Autodesk Inventor part; units mm, degrees
ref_plane "YZ Plane" through (0, 0, 0) normal (1, 0, 0) x (0, 1, 0)
ref_plane "XZ Plane" through (0, 0, 0) normal (0, 1, 0) x (-1, 0, 0)
ref_plane "XY Plane" through (0, 0, 0) normal (0, 0, 1) x (1, 0, 0)
sketch "Sketch1" plane through (0, 0, 0) normal (0, 0, 1) x (1, 0, 0)
  line L0 (0, 0) -> (0, 13.4062)
  line L1 (0, 0) -> (20.3742, 0)
  circle A0 centre (9.525, 12.7) radius 9.525 construction
  circle A1 centre (9.525, 12.7) radius 3.2004
  line L2 (31.75, 0) -> (7.8407, 6.5775)
  arc A2 (3.3908, 14.3415) -> (7.8407, 6.5775) centre (9.525, 12.7) ccw
  line L3 (31.75, 0) -> (76.2, 0)
  line L4 (76.2, 0) -> (76.2, 25.4)
  line L5 (76.2, 25.4) -> (31.75, 25.4)
  line L6 (31.75, 25.4) -> (31.75, 57.15)
  line L7 (31.75, 57.15) -> (19.05, 57.15)
  line L8 (19.05, 57.15) -> (19.05, 69.85)
  line L9 (19.05, 69.85) -> (6.35, 69.85)
  line L10 (6.35, 69.85) -> (6.35, 25.4)
  line L11 (6.35, 25.4) -> (3.3908, 14.3415)
  circle A3 centre (12.7, 63.5) radius 2.4892
  line L12 (12.7, 69.85) -> (12.7, 63.5)
  circle A4 centre (44.45, 12.7) radius 2.4892
  circle A5 centre (57.15, 12.7) radius 2.4892
  circle A6 centre (69.85, 12.7) radius 2.4892
  circle A7 centre (19.05, 38.1) radius 2.4892
  circle A8 centre (19.05, 50.8) radius 2.4892
  line L13 (19.05, 50.8) -> (19.05, 38.1) construction
  arc A9 (31.75, 29.8901) -> (36.2401, 25.4) centre (33.9951, 27.6451) ccw
  circle A10 centre (31.2867, 27.5124) radius 0.4633 construction
  circle A11 centre (33.8624, 24.9367) radius 0.4633 construction
  line L14 (31.75, 25.4) -> (31.2867, 27.5124) construction
  line L15 (31.75, 25.4) -> (33.8624, 24.9367) construction
  point P0 (76.2, 12.7)
  dimension "d0" = 19.05
  dimension "d1" = 3.175
  dimension "d2" = 6.4008
  dimension "d6" = 12.7
  dimension "d7" = 25.4
  dimension "d8" = 4.9784
  dimension "d16" = 6.35
  dimension "d17" = 25.4
  dimension "d19" = 6.35
  dimension "d24" = 12.7
  dimension "d29" = 6.35
  dimension "d30" = 12.7
  dimension "d35" = 12.7
  dimension "d36" = 12.7
  dimension "d37" = 12.7
  dimension "d38" = 6.35
  dimension "d39" = 12.7
  dimension "d40" = 6.35
extrude "Extrusion1" add sketch "Sketch1" along normal blind 3.175 contours L2 A2 L11 L10 L9 L8 L7 L6 A9 L5 L4 L3
fillet "Fillet1" radius 3.175 8 edges at (6.35, 69.85, 1.5875) (19.05, 69.85, 1.5875) (76.2, 25.4, 1.5875) (76.2, 0, 1.5875) (6.35, 25.4, 1.5875) (31.75, 0, 1.5875) (31.75, 57.15, 1.5875) (19.05, 57.15, 1.5875)
equation "\"d24\" = d11"
properties part number "Bottom Bearing Plate (R4 - 0.25in Between Stages)" material "Aluminum 6061"
Work out the finished part from the listing and answer in its coordinate system (mm). A direction names the side the tool comes from. Coordinates: 2 decimals unless noted, no trailing zeros. Write each loop counter-clockwise with the first axis right and the second up, starting at its lowest first coordinate (ties: lowest second). Pieces come first, ordered by that corner, then holes. Notation, with made-up numbers: M -6,87.25 L 1,87.25 A22 ccw 1,106.25 Z; hole C 46.25,73.5 d8. An arc over 180 degrees is marked long. Write item = value, one per line.
1. The part is cut by section D-D (y = 45). Determine the outline of the cut face in (x, z) (3 decimals).
Solution:
outline = M 6.35,0 L 31.75,0 L 31.75,3.175 L 6.35,3.175 Z
2. The part is cut by section A-A (y = 63.5). Determine the outline of the cut face in (x, z) (3 decimals).
Solution:
outline = M 6.35,0 L 10.211,0 L 10.211,3.175 L 6.35,3.175 Z; M 15.189,0 L 19.05,0 L 19.05,3.175 L 15.189,3.175 Z
3. For faces 1 (the face through (6.35, 47, 2)), 2 (the face through (55, 25.4, 2)), 3 (the face through (18.51, 53.23, 1.57)), determine the directions among +Z, -Z, +X, -X, +Y, -Y from which every point of the face is accessible in a straight line to the end or side of a thin tool.
Solution:
face_1 = +Z, -Z, -X, +Y
face_2 = +Z, -Z, +X, +Y
face_3 = +Z, -Z
4. Determine the mould class of faces 4 (the face through (19.05, 63, 2)), 5 (the face through (9.108, 9.527, 1.565)), 6 (the face through (25, 57.15, 2)) for opening direction Y: released by +Y, released by -Y, zero draft, split by the parting line, or undercut.
Solution:
face_4 = zero draft
face_5 = undercut
face_6 = released by +Y
5. Flat-ended cylindrical pins translate along their axes: pin 1 (1 mm diameter, centred on y = 44, z = 2, fed in from +X); pin 2 (4.5 mm diameter, centred on x = 69.85, y = 12.7, fed in from +Z); pin 3 (5.5 mm diameter, centred on x = 19.05, y = 50.8, fed in from +Z) (3 decimals); pin 4 (1 mm diameter, centred on y = 64, z = 1, fed in from +X). Find the tip coordinate at first contact, or state that the pin passes through.
Solution:
pin_1 = 31.75
pin_2 = through
pin_3 = 3.175
pin_4 = 19.05
6. Straight lines are drawn through the part: line 1 (Y direction, x = 69.85, z = 0.7); line 2 (Y direction, x = 17.5, z = 2.85); line 3 (X direction, y = 32, z = 1.3). For each, find the intervals that lie inside material, in ascending order. Write a range as from..to.
Solution:
line_1 = 0..10.21, 15.19..25.4
line_2 = 3.92..36.15, 40.05..48.85, 52.75..69.4
line_3 = 6.35..31.75
7. The part is cut by section B-B (z = 1.65). State how many separate pieces and enclosed holes the cut face has, then the cut area to 3 significant figures.
Solution:
separate_pieces = 1
enclosed_holes = 7
area = 2,520 mm2
8. The part is cut by section C-C (x = 57.15). Determine the outline of the cut face in (y, z) (3 decimals).
Solution:
outline = M 0,0 L 10.211,0 L 10.211,3.175 L 0,3.175 Z; M 15.189,0 L 25.4,0 L 25.4,3.175 L 15.189,3.175 Z
